Geometry check sheet. Reference: the model listing, model coordinates, mm. Give positions to 0.01 mm unless a question says otherwise; leave off trailing zeros. Order: outer loops, then holes, each group sorted by start corner. A loop starts at its lowest first (then second) coordinate and runs counter-clockwise, first axis right, second up. Notation, with made-up numbers: M -38,-19.5 L -10,-19.5 A27 cw -10,10.5 Z; hole C 33,33.25 d2. An arc over 180 degrees is marked long. Answer as CSV lines item,"result".
from build123d import *

# Parameters (mm, degrees)
F0_W     = 1500
F0_H     = 2000
F1_DEPTH = 180
F2_W     = 1440
F2_H     = 200
F3_DEPTH = 150


with BuildPart() as f1:
    # F0 (on Front) → F1 (new body)
    with BuildSketch(Plane.XZ):
        with Locations((750, 1000)):
            Rectangle(F0_W, F0_H)
    extrude(amount=F1_DEPTH)

    # F2 (on face) → F3 (cut)
    with BuildSketch(Plane.XZ.offset(180)):
        with Locations((750, 1870)):
            Rectangle(F2_W, F2_H)
        with Locations((750, 1640)):
            Rectangle(F2_W, F2_H)
        with Locations((750, 1410)):
            Rectangle(F2_W, F2_H)
        with Locations((750, 1180)):
            Rectangle(F2_W, F2_H)
        with Locations((750, 950)):
            Rectangle(F2_W, F2_H)
        with Locations((750, 720)):
            Rectangle(F2_W, F2_H)
        with Locations((750, 490)):
            Rectangle(F2_W, F2_H)
        with Locations((750, 260)):
            Rectangle(F2_W, F2_H)
    extrude(amount=-F3_DEPTH, mode=Mode.SUBTRACT)


solid = f1.part
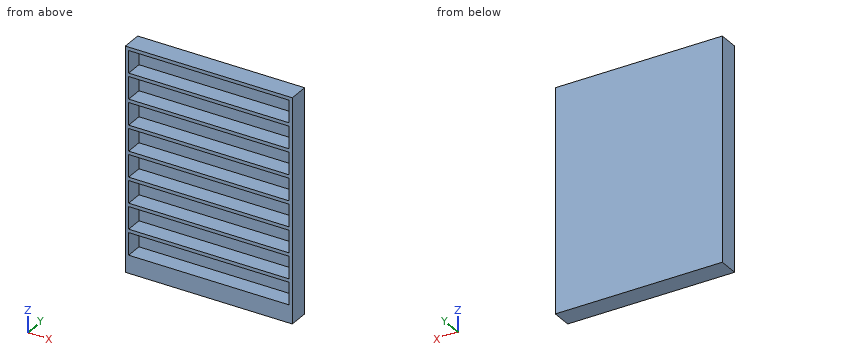
(1) Section check B-B on y = -155.5. State how many separate pieces and enclosed holes the cut face has, then the cut area to 3 significant figures.
The answers:
separate pieces,"1"
enclosed holes,"8"
area,"696,000 mm2"
(2) Gauge pin test, flat end, axial feed: P1, Ø1, axis at x = 994, z = 485.5, coming from the -Y side. Record the tip position at first contact, or that the pin passes through.
The answers:
P1,"stops at y = -30"
(3) Section check A-A on z = 1696. Enter the section's corners in (x, y).
The answers:
outline,"M 0,-180 L 30,-180 L 30,-30 L 1470,-30 L 1470,-180 L 1500,-180 L 1500,0 L 0,0 Z"
(4) Material ranges on line 1 (X direction, y = -75.5, z = 217); line 2 (Y direction, x = 373, z = 267), recorded low to high.
The answers:
line 1,"x = 0 to 30, 1470 to 1500"
line 2,"y = -30 to 0"
